from build123d import *

# Parameters (mm, degrees)
SKETCH1_W               = 5
SKETCH1_H               = 47
SKETCH2_W               = 18
SKETCH2_H               = 47
BOSS_EXTRUDE1_DEPTH     = 3.5
CUT_EXTRUDE1_DEPTH      = 47
CUT_EXTRUDE1_DEPTH_BACK = 47
SKETCH3_W               = 94
SKETCH3_H               = 94
SKETCH6_W               = 2
SKETCH6_H               = 53.4
CUT_EXTRUDE2_DEPTH      = 23.5
CUT_EXTRUDE2_DEPTH_BACK = 23.5


with BuildPart() as part:
    # Sketch1 → Revolve1 (revolve)
    with BuildSketch(Plane.XY, mode=Mode.PRIVATE) as revolve1_sk:
        with Locations((2.5, 0)):
            Rectangle(SKETCH1_W, SKETCH1_H)
    revolve(revolve1_sk.sketch.rotate(Axis((0, -23.5, 0), (0, 1, 0)), 270), axis=Axis((0, -23.5, 0), (0, 1, 0)))

    # Sketch2 → Boss-Extrude1 (add)
    with BuildSketch(Plane.XY.offset(-5)):
        with Locations((9, 0)):
            Rectangle(SKETCH2_W, SKETCH2_H)
    extrude(amount=BOSS_EXTRUDE1_DEPTH)

    # Sketch3 → Cut-Extrude1 (cut, two sides: drawn at the far end of the back side and taken through both)
    with BuildSketch(Plane.XY.offset(-CUT_EXTRUDE1_DEPTH_BACK)):
        Rectangle(SKETCH3_W, SKETCH3_H)
        Polygon((-5, 7.833333333), (5.25, 7.833333333), (5.25, -7.833333333), (-5, -7.833333333), (-5, -23.5), (18, -23.5), (18, 23.5), (-5, 23.5), align=None, mode=Mode.SUBTRACT)
    extrude(amount=CUT_EXTRUDE1_DEPTH + CUT_EXTRUDE1_DEPTH_BACK, mode=Mode.SUBTRACT)

    # Sketch4 → Revolve2 (revolve)
    with BuildSketch(Plane.XY, mode=Mode.PRIVATE) as revolve2_sk:
        Polygon((0, 25.2), (4, 25.2), (4, 24.35), (4.5, 24.35), (4.5, 23.5), (0, 23.5), align=None)
    revolve(revolve2_sk.sketch.rotate(Axis((0, 23.5, 0), (0, 1, 0)), 270), axis=Axis((0, 23.5, 0), (0, 1, 0)))

    # Sketch5 → Revolve3 (revolve)
    with BuildSketch(Plane.XY, mode=Mode.PRIVATE) as revolve3_sk:
        Polygon((0, -23.5), (4.5, -23.5), (4.5, -24.35), (4, -24.35), (4, -25.2), (0, -25.2), align=None)
    revolve(revolve3_sk.sketch.rotate(Axis((0, -25.2, 0), (0, 1, 0)), 270), axis=Axis((0, -25.2, 0), (0, 1, 0)))

    # Sketch6 → Cut-Revolve1 (revolve, cut)
    with BuildSketch(Plane.XY, mode=Mode.PRIVATE) as cut_revolve1_sk:
        with Locations((1, 0)):
            Rectangle(SKETCH6_W, SKETCH6_H)
    revolve(cut_revolve1_sk.sketch.rotate(Axis((0, -26.7, 0), (0, 1, 0)), 270), axis=Axis((0, -26.7, 0), (0, 1, 0)), mode=Mode.SUBTRACT)

    # Sketch7 → Cut-Revolve2 (revolve, cut)
    with BuildSketch(Plane(origin=(10.5, 0, 0), x_dir=(0, 0, -1), z_dir=(1, 0, 0)), mode=Mode.PRIVATE) as cut_revolve2_sk:
        Polygon((5, -12.5), (5, -15.25), (4.25, -15.25), (1.5, -18), (1.5, -12.5), align=None)
    revolve(cut_revolve2_sk.sketch.rotate(Axis((10.5, -12.5, -1.5), (0, 0, -1)), 90), axis=Axis((10.5, -12.5, -1.5), (0, 0, -1)), mode=Mode.SUBTRACT)

    # Sketch8 → Cut-Revolve3 (revolve, cut)
    with BuildSketch(Plane(origin=(10.5, 0, 0), x_dir=(0, 0, -1), z_dir=(1, 0, 0)), mode=Mode.PRIVATE) as cut_revolve3_sk:
        Polygon((5, 12.5), (5, 9.75), (4.25, 9.75), (1.5, 7), (1.5, 12.5), align=None)
    revolve(cut_revolve3_sk.sketch.rotate(Axis((10.5, 12.5, -1.5), (0, 0, -1)), 90), axis=Axis((10.5, 12.5, -1.5), (0, 0, -1)), mode=Mode.SUBTRACT)

    # Sketch9 → Cut-Extrude2 (cut, two sides: drawn at the far end of the back side and taken through both)
    with BuildSketch(Plane(origin=(0, 0, 0), x_dir=(1, 0, 0), z_dir=(0, 1, 0)).offset(-CUT_EXTRUDE2_DEPTH_BACK)):
        with BuildLine():
            Line((17, 1.5), (18, 1.5))
            Line((18, 1.5), (18, 2.5))
            ThreePointArc((18, 2.5), (17.707106781, 1.792893219), (17, 1.5))
        make_face()
    extrude(amount=CUT_EXTRUDE2_DEPTH + CUT_EXTRUDE2_DEPTH_BACK, mode=Mode.SUBTRACT)


solid = part.part
The model under review builds one solid part; all positions refer to its coordinate system, in mm. A direction names the side the tool comes from. Give positions to 0.01 mm unless a question says otherwise; leave off trailing zeros. Loops run counter-clockwise (first coordinate to the right, second up) from the corner with the lowest first, then second, coordinate; pieces in that order, holes last. Notation, with made-up numbers: (48, 50.5) -> (97, 50.5) arc R9 ccw to (97, 54.5) -> close; hole circle Ø11 at (13, -28). An arc over 180 degrees is marked (long way). Answer as a JSON object with one key per item and string values. Group by question number.
Q1. Take a section at B-B (x = 10.5). Write out the cut boundary in (y, z), plus the area to 3 significant figures.
Q2. Take a section at D-D (y = -19). Write out the cut boundary in (x, z), plus the area to 3 significant figures.
Q3. Wall thickness on line 1 along Y through (x, z) = (10.5, -4.7); line 2 along Y through (x, z) = (3.5, 2.75); line 3 along Y through (x, z) = (0, 2.25): over which ranges is each line inside the solid? List them lowest first.
Q4. Draft analysis for pull direction Z (two halves, no side actions). For faces 4 (the flat face through (2.3, 7.833, -0.1)), 5 (the cylindrical face through (-3.905, 24.769, -0.867)), 6 (the cylindrical face through (-2, -16, 0)), state which applies: pulls with the +Z half, pulls with the -Z half, needs draft (parallel to the pull), parting line crosses it, or undercut.
Q5. Insertion check: pin 1 (8 mm diameter, centred on x = 1.5, y = -0.5, fed in from -Z); pin 2 (9 mm diameter, centred on x = 10.5, y = -12.5, fed in from +Z); pin 3 (4 mm diameter, centred on x = 8, y = -7, fed in from +Z); pin 4 (1.8 mm diameter, centred on y = -2, z = -3, fed in from -X). Each pin has a flat end and moves straight along its axis. Give the tip position at first contact, or say it passes through.
Q6. Tool access review of faces 1 (the flat face through (5.25, 0, -3)), 2 (the cylindrical face through (-3.905, -24.781, -0.867)), 3 (the flat face through (-3, 24.35, 3)): name each direction out of +Z, -Z, +X, -X, +Y, -Y from which nothing blocks a thin tool from reaching the whole face with its end or side.
Q7. Take a section at C-C (z = 0). State how many separate pieces and enclosed holes the cut face has, plus the area to 3 significant figures.
Q8. Take a section at A-A (y = -12.5). Write out the cut boundary in (x, z), plus the area to 3 significant figures.
Answer below:
{
 "1": {"outline": "(-23.5, -5) -> (-15.25, -5) -> (-15.25, -4.25) -> (-18, -1.5) -> (-23.5, -1.5) -> close; (-9.75, -5) -> (9.75, -5) -> (9.75, -4.25) -> (7, -1.5) -> (-7, -1.5) -> (-9.75, -4.25) -> close; (15.25, -5) -> (23.5, -5) -> (23.5, -1.5) -> (18, -1.5) -> (15.25, -4.25) -> close", "area": "111 mm2"},
 "2": {"outline": "(0, -5) -> (18, -5) -> (18, -2.5) arc R1 ccw to (17, -1.5) -> (4.77, -1.5) arc R5 ccw (long way) to start; hole circle Ø4 at (0, 0)", "area": "117 mm2"},
 "3": {"line 1": "y = -23.5 to -15.25, -9.75 to 9.75, 15.25 to 23.5", "line 2": "y = -24.35 to -7.83, 7.83 to 24.35", "line 3": "y = -25.2 to -7.83, 7.83 to 25.2"},
 "4": {"face 4": "needs draft", "face 5": "parting line crosses it", "face 6": "undercut"},
 "5": {"pin 1": "stops at z = -5", "pin 2": "stops at z = -2.5", "pin 3": "stops at z = -1.5", "pin 4": "stops at x = 5.25"},
 "6": {"face 1": "+Z, -Z, -X", "face 2": "-Y", "face 3": "+Y"},
 "7": {"separate pieces": "4", "enclosed holes": "0", "area": "203 mm2"},
 "8": {"outline": "(0, -5) -> (7.75, -5) -> (7.75, -4.25) -> (5, -1.5) -> (4.77, -1.5) arc R5 ccw (long way) to start; (13.25, -5) -> (18, -5) -> (18, -2.5) arc R1 ccw to (17, -1.5) -> (16, -1.5) -> (13.25, -4.25) -> close; hole circle Ø4 at (0, 0)", "area": "89.7 mm2"}
}
